from build123d import *

# Parameters (mm, degrees)
SKETCH1_W           = 38
SKETCH1_H           = 38
BOSS_EXTRUDE1_DEPTH = 7
SKETCH2_R           = 4.25
CUT_EXTRUDE1_DEPTH  = 7
SKETCH3_R           = 11.25
CUT_EXTRUDE2_DEPTH  = 3.1
SKETCH5_R           = 1.75
CUT_EXTRUDE3_DEPTH  = 27
SKETCH6_R           = 2.75
SKETCH6_R_2         = 1.75
CUT_EXTRUDE14_DEPTH = 3.5


with BuildPart() as part:
    # Sketch1 → Boss-Extrude1 (new body)
    with BuildSketch(Plane(origin=(0, 0, 0), x_dir=(1, 0, 0), z_dir=(0, 1, 0))):
        Rectangle(SKETCH1_W, SKETCH1_H)
    extrude(amount=BOSS_EXTRUDE1_DEPTH)

    # Sketch2 → Cut-Extrude1 (cut)
    with BuildSketch(Plane(origin=(0, 7, 0), x_dir=(1, 0, 0), z_dir=(0, 1, 0))):
        with BuildLine():
            ThreePointArc((-13.75, 15.5), (-16.737436867, 16.737436867), (-15.5, 13.75))
            Line((-15.5, 13.75), (-15.5, 15.5))
            Line((-15.5, 15.5), (-13.75, 15.5))
        make_face()
        with BuildLine():
            Line((-15.5, 15.5), (-15.5, 13.75))
            ThreePointArc((-15.5, 13.75), (-14.262563133, 14.262563133), (-13.75, 15.5))
            Line((-13.75, 15.5), (-15.5, 15.5))
        make_face()
        with BuildLine():
            ThreePointArc((13.75, 15.5), (14.262563133, 14.262563133), (15.5, 13.75))
            Line((15.5, 13.75), (15.5, 15.5))
            Line((15.5, 15.5), (13.75, 15.5))
        make_face()
        with BuildLine():
            Line((15.5, 15.5), (15.5, 13.75))
            ThreePointArc((15.5, 13.75), (16.737436867, 14.262563133), (17.25, 15.5))
            ThreePointArc((17.25, 15.5), (15.5, 17.25), (13.75, 15.5))
            Line((13.75, 15.5), (15.5, 15.5))
        make_face()
        with BuildLine():
            ThreePointArc((15.5, -13.75), (14.262563133, -14.262563133), (13.75, -15.5))
            Line((13.75, -15.5), (15.5, -15.5))
            Line((15.5, -15.5), (15.5, -13.75))
        make_face()
        with BuildLine():
            Line((15.5, -15.5), (13.75, -15.5))
            ThreePointArc((13.75, -15.5), (15.5, -17.25), (17.25, -15.5))
            ThreePointArc((17.25, -15.5), (16.737436867, -14.262563133), (15.5, -13.75))
            Line((15.5, -13.75), (15.5, -15.5))
        make_face()
        with BuildLine():
            ThreePointArc((-15.5, -13.75), (-16.737436867, -16.737436867), (-13.75, -15.5))
            Line((-13.75, -15.5), (-15.5, -15.5))
            Line((-15.5, -15.5), (-15.5, -13.75))
        make_face()
        with BuildLine():
            Line((-15.5, -15.5), (-13.75, -15.5))
            ThreePointArc((-13.75, -15.5), (-14.262563133, -14.262563133), (-15.5, -13.75))
            Line((-15.5, -13.75), (-15.5, -15.5))
        make_face()
        Circle(SKETCH2_R)
    extrude(amount=-CUT_EXTRUDE1_DEPTH, mode=Mode.SUBTRACT)

    # Sketch3 → Cut-Extrude2 (cut)
    with BuildSketch(Plane(origin=(0, 7, 0), x_dir=(1, 0, 0), z_dir=(0, 1, 0))):
        Circle(SKETCH3_R)
    extrude(amount=-CUT_EXTRUDE2_DEPTH, mode=Mode.SUBTRACT)

    # Sketch5 → Cut-Extrude3 (cut)
    with BuildSketch(Plane(origin=(0, 7, 0), x_dir=(1, 0, 0), z_dir=(0, 1, 0))):
        with Locations((-9.899494937, 9.899494937)):
            Circle(SKETCH5_R)
        with Locations((9.899494937, 9.899494937)):
            Circle(SKETCH5_R)
        with Locations((9.899494937, -9.899494937)):
            Circle(SKETCH5_R)
        with Locations((-9.899494937, -9.899494937)):
            Circle(SKETCH5_R)
    extrude(amount=-CUT_EXTRUDE3_DEPTH, mode=Mode.SUBTRACT)

    # Sketch6 → Cut-Extrude14 (cut)
    with BuildSketch(Plane.XZ):
        with Locations((-9.899494937, 9.899494937)):
            Circle(SKETCH6_R)
        with Locations((-9.899494937, 9.899494937)):
            Circle(SKETCH6_R_2, mode=Mode.SUBTRACT)
        with Locations((9.899494937, 9.899494937)):
            Circle(SKETCH6_R)
        with Locations((9.899494937, 9.899494937)):
            Circle(SKETCH6_R_2, mode=Mode.SUBTRACT)
        with Locations((9.899494937, -9.899494937)):
            Circle(SKETCH6_R)
        with Locations((9.899494937, -9.899494937)):
            Circle(SKETCH6_R_2, mode=Mode.SUBTRACT)
        with Locations((-9.899494937, -9.899494937)):
            Circle(SKETCH6_R)
        with Locations((-9.899494937, -9.899494937)):
            Circle(SKETCH6_R_2, mode=Mode.SUBTRACT)
    extrude(amount=-CUT_EXTRUDE14_DEPTH, mode=Mode.SUBTRACT)


solid = part.part
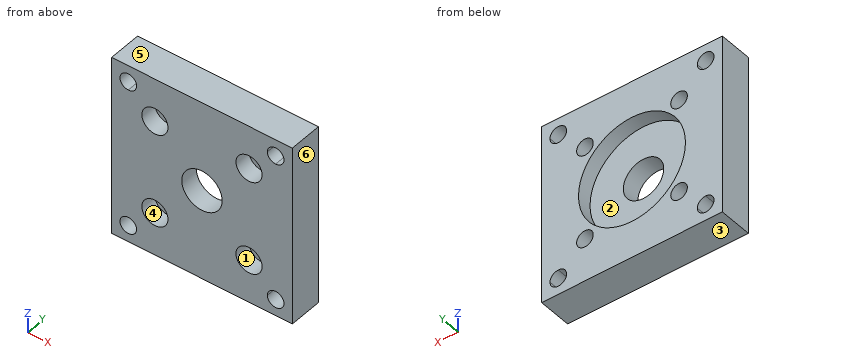
Part model, mm, in its own coordinate system. Face numbers are marked on the shaded views. A direction names the side the tool comes from. Round coordinates to 2 decimals unless told otherwise and drop trailing zeros. Loops run counter-clockwise (first coordinate to the right, second up) from the corner with the lowest first, then second, coordinate; pieces in that order, holes last. Notation, with made-up numbers: (89.25, 5.5) - (143.25, 5.5) arc R7 cw to (143.25, 10.5) - close; hole circle Ø7 at (22.5, 11.25). An arc over 180 degrees is marked (long way). Answer as a JSON object with one key per item and string values.
Item 1: Band-saw the part on C-C on x = 9. List the corners of the cut face in (y, z).
Output:
{"outline": "(0, -19) - (7, -19) - (7, -11.4) - (3.5, -11.4) - (3.5, -12.5) - (0, -12.5) - close; (0, -7.3) - (3.5, -7.3) - (3.5, -8.4) - (7, -8.4) - (7, -6.75) - (3.9, -6.75) - (3.9, 6.75) - (7, 6.75) - (7, 8.4) - (3.5, 8.4) - (3.5, 7.3) - (0, 7.3) - close; (0, 12.5) - (3.5, 12.5) - (3.5, 11.4) - (7, 11.4) - (7, 19) - (0, 19) - close"}
Item 2: Band-saw the part on D-D on z = 15. List the corners of the cut face in (x, y).
Output:
{"outline": "(-19, 0) - (-17.18, 0) - (-17.18, 7) - (-19, 7) - close; (-13.82, 0) - (13.82, 0) - (13.82, 7) - (-13.82, 7) - close; (17.18, 0) - (19, 0) - (19, 7) - (17.18, 7) - close"}
Item 3: Pull direction Z, two halves, no side cores. Call the marked faces 4, 5 and 6: pulls with the +Z half, pulls with the -Z half, needs draft (parallel to the pull), parting line crosses it, or undercut.
Output:
{"face 4": "undercut", "face 5": "pulls with the +Z half", "face 6": "needs draft"}
Item 4: Band-saw the part on A-A on z = 0. List the corners of the cut face in (x, y).
Output:
{"outline": "(-19, 0) - (-4.25, 0) - (-4.25, 3.9) - (-11.25, 3.9) - (-11.25, 7) - (-19, 7) - close; (4.25, 0) - (19, 0) - (19, 7) - (11.25, 7) - (11.25, 3.9) - (4.25, 3.9) - close"}
Item 5: Pin check, flat tips, straight feed: pin 1 (4.5 mm diameter, centred on x = -15.5, z = -15.5, fed in from +Y); pin 2 (5 mm diameter, centred on x = 9.9, z = -9.9, fed in from -Y); pin 3 (10 mm diameter, centred on x = 0, z = 0, fed in from +Y). Stop position of each tip, or through.
Output:
{"pin 1": "y = 7", "pin 2": "y = 3.5", "pin 3": "y = 3.9"}
Item 6: Tool access for the marked faces 1, 2 and 3: list every direction of +Z, -Z, +X, -X, +Y, -Y with a clear straight run to the whole face (end or side of a thin tool).
Output:
{"face 1": "-Y", "face 2": "+Y", "face 3": "-Z, +X, -X, +Y, -Y"}
Item 7: Band-saw the part on B-B on x = 0. List the corners of the cut face in (y, z).
Output:
{"outline": "(0, -19) - (7, -19) - (7, -11.25) - (3.9, -11.25) - (3.9, -4.25) - (0, -4.25) - close; (0, 4.25) - (3.9, 4.25) - (3.9, 11.25) - (7, 11.25) - (7, 19) - (0, 19) - close"}
Item 8: Wall check: L1, parallel to X at y = 4.5, z = -15.5; L2, parallel to X at y = 4.25, z = -8.5. Give the ranges that are in metal, low to high.
Output:
{"L1": "-19 to -17.25, -13.75 to 13.75, 17.25 to 19", "L2": "-19 to -10.95, -8.85 to -7.37, 7.37 to 8.85, 10.95 to 19"}
